Verification items for the finished model (mm, model axes). A direction names the side the tool comes from. Coordinates: 2 decimals unless noted, no trailing zeros. Write each loop counter-clockwise with the first axis right and the second up, starting at its lowest first coordinate (ties: lowest second). Pieces come first, ordered by that corner, then holes. Notation, with made-up numbers: (82.25, 29) -> (131.25, 29) arc R24 ccw to (131.25, 66) -> close; hole circle Ø7 at (35.5, 35). An arc over 180 degrees is marked (long way). Answer in a Markdown table with one row per item.
```python
from build123d import *

# Parameters (mm, degrees)
F1_DEPTH  = 152.4
F2_W      = 254
F2_H      = 148.59
F3_DEPTH  = 504.19
F4_R      = 12.7
F5_W      = 3.81
F5_H      = 135.89
F6_DEPTH  = 50.8
F7_W      = 3.81
F7_H      = 135.89
F8_DEPTH  = 50.8
F10_DEPTH = 25.4
F12_DEPTH = 25.4


with BuildPart() as f1:
    # F0 (on Top) → F1 (new body)
    with BuildSketch(Plane.XY):
        Polygon((-88.9, -508), (165.1, -508), (165.1, -444.5), (76.2, -444.5), (76.2, -342.9), (165.1, -342.9), (165.1, -279.4), (76.2, -279.4), (76.2, 0), (0, 0), (0, -279.4), (-88.9, -279.4), (-88.9, -342.9), (0, -342.9), (0, -444.5), (-88.9, -444.5), align=None)
    extrude(amount=F1_DEPTH)

    # F2 (on face) → F3 (cut)
    with BuildSketch(Plane.XZ.offset(508)):
        with Locations((38.1, 74.295)):
            Rectangle(F2_W, F2_H)
    extrude(amount=-F3_DEPTH, mode=Mode.SUBTRACT)

    # F4
    f4_edges = [f1.edges().sort_by_distance(p)[0] for p in [
        (38.1, 0, 152.4),
        (38.1, -3.81, 148.59),
    ]]
    fillet(f4_edges, radius=F4_R)

    # F5 (on face) → F6 (join)
    with BuildSketch(Plane.YZ.offset(76.2)):
        with Locations((-1.905, 67.945)):
            Rectangle(F5_W, F5_H)
    extrude(amount=F6_DEPTH)

    # F7 (on face) → F8 (join)
    with BuildSketch(Plane(origin=(0, 0, 0), x_dir=(0, -1, 0), z_dir=(-1, 0, 0))):
        with Locations((1.905, 67.945)):
            Rectangle(F7_W, F7_H)
    extrude(amount=F8_DEPTH)

    # F9 (on face) → F10 (join)
    with BuildSketch(Plane.YZ.offset(76.2)):
        Polygon((-393.7, 148.59), (-3.81, 0), (-3.81, 4.07731), (-383.001416, 148.59), align=None)
    extrude(amount=-F10_DEPTH)

    # F11 (on face) → F12 (join)
    with BuildSketch(Plane(origin=(0, 0, 0), x_dir=(0, -1, 0), z_dir=(-1, 0, 0))):
        Polygon((3.81, 0), (393.7, 148.59), (383.001416, 148.59), (3.81, 4.07731), align=None)
    extrude(amount=-F12_DEPTH)


solid = f1.part
```
1. Sectioned sample at A-A, the plane x = 149. Record the cut outline in (y, z), and give its area (3 significant figures).
Findings below:
| item | result |
|---|---|
| outline | (-508, 148.59) -> (-444.5, 148.59) -> (-444.5, 152.4) -> (-508, 152.4) -> close; (-342.9, 148.59) -> (-279.4, 148.59) -> (-279.4, 152.4) -> (-342.9, 152.4) -> close |
| area | 484 mm² |
2. Sectioned sample at D-D, the plane y = -471.5. Record the cut outline in (x, z).
Findings below:
| item | result |
|---|---|
| outline | (-88.9, 148.59) -> (165.1, 148.59) -> (165.1, 152.4) -> (-88.9, 152.4) -> close |
3. Material ranges on probe 1 along Z at (x, y) = (33, -209); probe 2 along Y at (x, z) = (-38, 64.5); probe 3 along Z at (x, y) = (75, -140), recorded low to high. Write a range as from..to.
Findings below:
| item | result |
|---|---|
| probe 1 | z = 148.59..152.4 |
| probe 2 | y = -3.81..0 |
| probe 3 | z = 51.9..55.98, 148.59..152.4 |
4. Sectioned sample at C-C, the plane z = 28.5. Record the cut outline in (x, y), and give its area (3 significant figures).
Findings below:
| item | result |
|---|---|
| outline | (-50.8, -3.81) -> (127, -3.81) -> (127, 0) -> (-50.8, 0) -> close; (0, -78.59) -> (25.4, -78.59) -> (25.4, -67.89) -> (0, -67.89) -> close; (50.8, -78.59) -> (76.2, -78.59) -> (76.2, -67.89) -> (50.8, -67.89) -> close |
| area | 1,220 mm² |
5. Access from +Z, -Z, +X, -X, +Y, -Y to the whole of each face (thin tool, end or side, straight path). Record for faces 1 (the face through (0, -256, 99)), 2 (the face through (76.2, -258, 99)), 3 (the face through (37.57, -3.82, 148.78)), 4 (the face through (38.63, -7.63, 144.97)), 5 (the face through (63.678, -201.484, 75.335)).
Findings below:
| item | result |
|---|---|
| face 1 | -Z, -X |
| face 2 | -Z, +X |
| face 3 | +Z, +X, -X, +Y |
| face 4 | +X, -X |
| face 5 | -Z, +X, -X, -Y |
6. Sectioned sample at B-B, the plane y = -307.5. Record the cut outline in (x, z).
Findings below:
| item | result |
|---|---|
| outline | (-88.9, 148.59) -> (165.1, 148.59) -> (165.1, 152.4) -> (-88.9, 152.4) -> close; (0, 115.74) -> (25.4, 115.74) -> (25.4, 119.82) -> (0, 119.82) -> close; (50.8, 115.74) -> (76.2, 115.74) -> (76.2, 119.82) -> (50.8, 119.82) -> close |
7. Go/stop test with flat-tipped pins: pin 1 (4 mm diameter, centred on x = -28, y = -2.5, fed in from +Z); pin 2 (13 mm diameter, centred on y = -132, z = 142.5, fed in from +X); pin 3 (1 mm diameter, centred on x = 110, y = -295.5, fed in from -Z). Record where each tip stops, or that it passes through.
Findings below:
| item | result |
|---|---|
| pin 1 | stops at z = 135.89 |
| pin 2 | stops at x = 76.2 |
| pin 3 | stops at z = 148.59 |
8. Release check for a two-part mould opening along X. For faces 6 (the face through (25.4, -198, 75)), 7 (the face through (76.2, -140, 150)), 8 (the face through (12.522, -196.026, 73.255)) record: released by +X, released by -X, zero draft, split by the parting line, or undercut.
Findings below:
| item | result |
|---|---|
| face 6 | undercut |
| face 7 | released by +X |
| face 8 | zero draft |
